CAD build for the part. Positions are in the model's coordinates, mm. A direction names the side the tool comes from. Coordinates: 2 decimals unless noted, no trailing zeros.
```python
from build123d import *

# Parameters (mm, degrees)
SKETCH1_R           = 50
SKETCH1_R_2         = 40
EXTRUDE_THIN1_DEPTH = 10
SKETCH2_R           = 7.5
SKETCH2_R_2         = 2.5
BOSS_EXTRUDE1_DEPTH = 6
BOSS_EXTRUDE4_DEPTH = 3
FILLET4_R           = 8
FILLET2_R           = 3
FILLET3_R           = 2


# Some blends are built 0.0001 mm under size
with BuildPart() as part:
    # Sketch1 → Extrude-Thin1 (new body)
    with BuildSketch(Plane.XY):
        Circle(SKETCH1_R)
        Circle(SKETCH1_R_2, mode=Mode.SUBTRACT)
    extrude(amount=EXTRUDE_THIN1_DEPTH)



with BuildPart() as body_2:
    # Sketch2 → Boss-Extrude1 (new body)
    with BuildSketch(Plane.XY):
        Circle(SKETCH2_R)
        Circle(SKETCH2_R_2, mode=Mode.SUBTRACT)
    extrude(amount=BOSS_EXTRUDE1_DEPTH)


with BuildPart() as part_1:
    add(part.part)

    add(body_2.part)  # Boss-Extrude4 merges body 2
    # Sketch3 → Boss-Extrude4 (add)
    with BuildSketch(Plane.XY):
        with BuildLine():
            ThreePointArc((-3, 6.873863542), (-1.532322328, 7.341797347), (0, 7.5))
            Line((0, 7.5), (0, 40))
            ThreePointArc((0, 40), (-0.75, 39.992968132), (-1.499736305, 39.971875))
            Line((-1.499736305, 39.971875), (-3, 6.873863542))
        make_face()
        with BuildLine():
            Line((0, 40), (0, 7.5))
            ThreePointArc((0, 7.5), (1.532322328, 7.341797347), (3, 6.873863542))
            Line((3, 6.873863542), (1.499736305, 39.971875))
            ThreePointArc((1.499736305, 39.971875), (0.75, 39.992968132), (0, 40))
        make_face()
        with BuildLine():
            Line((4.45294045, -6.035007983), (33.866791034, -21.284747239))
            ThreePointArc((33.866791034, -21.284747239), (34.641016151, -20), (35.366527339, -18.687127761))
            Line((35.366527339, -18.687127761), (7.45294045, -0.83885556))
            ThreePointArc((7.45294045, -0.83885556), (6.495190528, -3.75), (4.45294045, -6.035007983))
        make_face()
        with BuildLine():
            ThreePointArc((-35.366527339, -18.687127761), (-34.641016151, -20), (-33.866791034, -21.284747239))
            Line((-33.866791034, -21.284747239), (-4.45294045, -6.035007983))
            ThreePointArc((-4.45294045, -6.035007983), (-6.495190528, -3.75), (-7.45294045, -0.83885556))
            Line((-7.45294045, -0.83885556), (-35.366527339, -18.687127761))
        make_face()
    extrude(amount=BOSS_EXTRUDE4_DEPTH)

    # Fillet4
    # the kernel refuses this fillet: 8 mm, written as the material it adds along each edge
    with BuildSketch(Plane(origin=(-3, 6.873863542, 0), x_dir=(-0.829854636614874, -0.5579796430774114, 0), z_dir=(0, 0, 1)), Plane(origin=(7.45294045, -0.83885556, 0), x_dir=(-0.06829722739215581, 0.9976650182954919, 0), z_dir=(0, 0, 1)), Plane(origin=(-4.45294045, -6.035007983, 0), x_dir=(0.8981518640070405, -0.43968537521809675, 0), z_dir=(0, 0, 1))) as fillet4_piece_1:
        with BuildLine():
            CenterArc((4.127463516, -7.870129559), FILLET4_R, 100.338012957, 43.150474146)
            Line((-2.302435059, -3.110255158), (0, 0))
            ThreePointArc((0, 0), (1.345912016, -0.121753539), (2.691824032, 0))
        make_face()
    extrude(amount=3)
    with BuildSketch(Plane(origin=(3, 6.873863542, 0), x_dir=(0.8298546366148741, -0.5579796430774113, 0), z_dir=(0, 0, 1)), Plane(origin=(4.45294045, -6.035007983, 0), x_dir=(-0.8981518640070573, -0.4396853752180626, 0), z_dir=(0, 0, 1)), Plane(origin=(-7.45294045, -0.83885556, 0), x_dir=(0.06829722739219261, 0.9976650182954894, 0), z_dir=(0, 0, 1))) as fillet4_piece_2:
        with BuildLine():
            CenterArc((4.127463516, 7.870129559), FILLET4_R, 216.511512897, 43.150474146)
            Line((-2.302435059, 3.110255158), (0, 0))
            ThreePointArc((0, 0), (1.345912016, 0.121753539), (2.691824032, 0))
        make_face()
    extrude(amount=3)
    with BuildSketch(Plane(origin=(1.499736305, 39.971875, 0), x_dir=(0.04528141614846467, -0.9989742706154096, 0), z_dir=(0, 0, 1)), Plane(origin=(33.866791034, -21.284747239, 0), x_dir=(-0.8877778041541985, 0.46027227860381686, 0), z_dir=(0, 0, 1)), Plane(origin=(-35.366527339, -18.687127761, 0), x_dir=(0.8424963880057403, 0.5387019920116138, 0), z_dir=(0, 0, 1))) as fillet4_piece_3:
        with BuildLine():
            CenterArc((9.927616813, 8), FILLET4_R, 159.305768692, 110.694231308)
            ThreePointArc((2.443779894, 10.827045272), (0.84452181, 5.49869866), (0, 0))
            Line((0, 0), (9.927616813, 0))
        make_face()
    extrude(amount=3)
    with BuildSketch(Plane(origin=(-1.499736305, 39.971875, 0), x_dir=(-0.04528141614846486, -0.9989742706154096, 0), z_dir=(0, 0, 1)), Plane(origin=(35.366527339, -18.687127761, 0), x_dir=(-0.8424963880057321, 0.5387019920116268, 0), z_dir=(0, 0, 1)), Plane(origin=(-33.866791034, -21.284747239, 0), x_dir=(0.8877778041542049, 0.4602722786038045, 0), z_dir=(0, 0, 1))) as fillet4_piece_4:
        with BuildLine():
            CenterArc((9.927616813, -8), FILLET4_R, 90, 110.694231308)
            ThreePointArc((2.443779894, -10.827045272), (0.84452181, -5.49869866), (0, 0))
            Line((0, 0), (9.927616813, 0))
        make_face()
    extrude(amount=3)

    # Fillet2
    fillet2_edges = [part_1.edges().sort_by_distance(p)[0] for p in [
        (-7.5, 0, 6),
    ]]
    fillet(fillet2_edges, radius=FILLET2_R - 0.0001)  # a hair under: the kernel refuses the full size

    # Fillet3
    fillet3_edges = [part_1.edges().sort_by_distance(p)[0] for p in [
        (-50, 0, 0),
        (-50, 0, 10),
        (-40, 0, 10),
    ]]
    fillet(fillet3_edges, radius=FILLET3_R)


solid = part_1.part
```
Item 1: Two-plate mould, pull along X, no slides. Class faces 1 (the cylindrical face through (5.185, 36.85, 1.479)), 2 (the cylindrical face through (47.69, 15.02, 4.96)), 3 (the flat face through (-0.2, -42.4, 10)): +X half, -X half, draft (parallel to the pull), parting line (faces both ways), or undercut.
Item 2: Flat gauge pins, fed straight in: pin 1 Ø4 at (y, z) = (37.5, 5) entering from -X; pin 2 Ø5 at (x, y) = (6.5, 8.5) entering from +Z; pin 3 Ø6 at (x, z) = (27, 8.5) entering from -Y; pin 4 Ø6.5 at (x, y) = (0, 0) entering from +Z. Where does each tip first touch, or does it go through?
Item 3: Saw through at A-A, the plane x = 0. State how many separate pieces and enclosed holes the cut face has, and give its area (3 significant figures).
Item 4: Wall check: line 1 along Y through (x, z) = (0, 3.05); line 2 along Y through (x, z) = (0, 2.75); line 3 along X through (y, z) = (10.5, 1.25). Give the ranges that are in metal, low to high.
Item 5: Which spindle directions (+Z, -Z, +X, -X, +Y, -Y) get a long thin tool onto all of the face, cutting with end or side? Do faces 4 (the flat face through (-18.744, -8.058, 1.479)), 5 (the cylindrical face through (38.153, 12.015, 3.944)). Say none if no direction does.
Working result:
1. face 1: undercut
1. face 2: parting line
1. face 3: draft
2. pin 1: stops at x = -35.21
2. pin 2: passes through
2. pin 3: stops at y = -43.85
2. pin 4: stops at z = 6
3. separate pieces: 3
3. enclosed holes: 0
3. area: 348 mm2
4. line 1: y = -50 to -40, -7.5 to -2.5, 2.5 to 7.5, 40 to 50
4. line 2: y = -50 to -40, -7.5 to -2.5, 2.5 to 50
4. line 3: x = -48.74 to -38.6, -2.84 to 2.84, 38.6 to 48.74
5. face 4: +Z, -Z
5. face 5: +Z
